Verification items for the finished model (mm, model axes). A direction names the side the tool comes from. Round coordinates to 2 decimals unless told otherwise and drop trailing zeros. Write each loop counter-clockwise with the first axis right and the second up, starting at its lowest first coordinate (ties: lowest second). Pieces come first, ordered by that corner, then holes. Notation, with made-up numbers: (46.25, -18.75) - (74.25, -18.75) arc R17 cw to (74.25, -9.75) - close; hole circle Ø8 at (85, 63). An arc over 180 degrees is marked (long way). Answer as a JSON object with one key per item and string values.
```python
from build123d import *

# Parameters (mm, degrees)
F0_R     = 177.8
F1_DEPTH = 19.05
F2_R     = 12.7
F3_T     = -0.6985
F5_DEPTH = 12.7


with BuildPart() as f1:
    # F0 (on Top) → F1 (new body, symmetric)
    with BuildSketch(Plane.XY):
        Circle(F0_R)
    extrude(amount=F1_DEPTH, both=True)

    # F2
    f2_edges = [f1.edges().sort_by_distance(p)[0] for p in [
        (-177.8, 0, -19.05),
    ]]
    fillet(f2_edges, radius=F2_R)

    # F3
    f3_openings = [f1.faces().sort_by_distance(p)[0] for p in [
        (0, 0, 19.05),
    ]]
    offset(amount=F3_T, openings=f3_openings)

    # F4 (on face) → F5 (cut, symmetric)
    with BuildSketch(Plane(origin=(0, 0, -19.05), x_dir=(1, 0, 0), z_dir=(0, 0, -1))):
        with BuildLine():
            Line((12.7, -25.399946), (12.699786, 25.326312))
            ThreePointArc((12.699786, 25.326312), (0.036844, 38.099947), (-12.7, 25.4))
            Line((-12.7, 25.4), (-12.7, -25.4))
            ThreePointArc((-12.7, -25.4), (2.7e-05, -38.1), (12.7, -25.399946))
        make_face()
    extrude(amount=F5_DEPTH, both=True, mode=Mode.SUBTRACT)


solid = f1.part
```
Q1. Set-up check for faces 1 (the flat face through (34, 2, -18.352)), 2 (the cylindrical face through (-0.279, 38.097, -18.706)): record each of +Z, -Z, +X, -X, +Y, -Y from which the full face is reachable in a straight line by a thin tool's end or side.
Geometry check:
{"face 1": "+Z", "face 2": "+Z, -Z"}
Q2. Material ranges on line 1 along Y through (x, z) = (0, 9); line 2 along X through (y, z) = (-3.5, 17); line 3 along Z through (x, y) = (-46, -35.5), recorded low to high. Write a range as [from, to].
Geometry check:
{"line 1": "y = [-177.8, -177.1], [177.1, 177.8]", "line 2": "x = [-177.77, -177.07], [177.07, 177.77]", "line 3": "z = [-19.05, -18.35]"}
Q3. Section check C-C, the plane z = 13.5. Record the cut outline in (x, y), then the cut area to 3 significant figures.
Geometry check:
{"outline": "circle Ø355.6 at (0, 0); hole circle Ø354.2 at (0, 0)", "area": "779 mm2"}
Q4. Section check B-B, the plane y = 0. Record the cut outline in (x, z).
Geometry check:
{"outline": "(-177.8, -6.35) arc R12.7 ccw to (-165.1, -19.05) - (-12.7, -19.05) - (-12.7, -18.35) - (-165.1, -18.35) arc R12 cw to (-177.1, -6.35) - (-177.1, 19.05) - (-177.8, 19.05) - close; (12.7, -19.05) - (165.1, -19.05) arc R12.7 ccw to (177.8, -6.35) - (177.8, 19.05) - (177.1, 19.05) - (177.1, -6.35) arc R12 cw to (165.1, -18.35) - (12.7, -18.35) - close"}
Q5. Release check for a two-part mould opening along Y. For faces 3 (the cylindrical face through (169.59, 53.41, 6.53)), 4 (the flat face through (34, 2, -19.05)), 5 (the cylindrical face through (0.317, -38.096, -18.706)) record: released by +Y, released by -Y, zero draft, split by the parting line, or undercut.
Geometry check:
{"face 3": "split by the parting line", "face 4": "zero draft", "face 5": "undercut"}
Q6. Section check A-A, the plane x = 0. Record the cut outline in (y, z).
Geometry check:
{"outline": "(-177.8, -6.35) arc R12.7 ccw to (-165.1, -19.05) - (-38.1, -19.05) - (-38.1, -18.35) - (-165.1, -18.35) arc R12 cw to (-177.1, -6.35) - (-177.1, 19.05) - (-177.8, 19.05) - close; (38.1, -19.05) - (165.1, -19.05) arc R12.7 ccw to (177.8, -6.35) - (177.8, 19.05) - (177.1, 19.05) - (177.1, -6.35) arc R12 cw to (165.1, -18.35) - (38.1, -18.35) - close"}
Q7. Gauge pin test, flat ends, axial feed: P1, Ø6, axis at y = 116.5, z = 15, coming from the -X side; P2, Ø12, axis at x = 58.5, y = -75.5, coming from the +Z side; P3, Ø10, axis at y = 29.5, z = 3, coming from the -X side. Record the tip position at first contact, or that the pin passes through.
Geometry check:
{"P1": "stops at x = -136.86", "P2": "stops at z = -18.35", "P3": "stops at x = -176.1"}
Q8. Section check D-D, the plane z = -14. Record the cut outline in (x, y), then the cut area to 3 significant figures.
Geometry check:
{"outline": "circle Ø350.47 at (0, 0); hole circle Ø348.69 at (0, 0)", "area": "978 mm2"}
